Read the model definition and answer for the solid it produces. Units are mm, in the model's axes. A direction names the side the tool comes from. Round coordinates to 2 decimals unless told otherwise and drop trailing zeros. Write each loop counter-clockwise with the first axis right and the second up, starting at its lowest first coordinate (ties: lowest second). Pieces come first, ordered by that corner, then holes. Notation, with made-up numbers: (28, 56.25) - (39, 56.25) arc R29 cw to (39, 81.25) - close; hole circle Ø7 at (-14, 82). An arc over 180 degrees is marked (long way). Answer as CSV lines item,"result". Start each with the question number.
1) Find section C-C on y = -10. Determine the outline of the cut face in (x, z).
2) Find section B-B on z = 14.75. Determine the outline of the cut face in (x, y), then the cut area to 3 significant figures.
3) Find section D-D on x = -8.5. Determine the outline of the cut face in (y, z), then the cut area to 3 significant figures.
4) Find section A-A on z = 8.5. Determine the outline of the cut face in (x, y), then the cut area to 3 significant figures.
5) For a pull along Y with two mould halves and no side action, classify faces 3 (the flat face through (-26, -12.186, 8)), 4 (the cylindrical face through (-26.3, -3.58, 10.36)), 5 (the flat face through (-26, 10, 0)) as +Y half, -Y half, draft (parallel to the pull), parting line (faces both ways), or undercut.
6) Consider line 1 along X through (y, z) = (17, 8); line 2 along X through (y, z) = (-2, 9.5); line 3 along Y through (x, z) = (-0.5, 9.5). Determine where each line is inside the solid, lowest interval first.
7) Each of these flat-tipped pins is pushed along its axis until it touches: pin 1 (1 mm diameter, centred on y = 3.5, z = 4.5, fed in from +X); pin 2 (4.5 mm diameter, centred on x = -5.28, z = 8, fed in from -Y); pin 3 (12 mm diameter, centred on x = -7, y = 5, fed in from +Z) (1 decimal); pin 4 (6.5 mm diameter, centred on y = -4.18, z = 8.45, fed in from -X). Where does it stop, or does it pass through?
8) Which of the six approach directions +Z, -Z, +X, -X, +Y, -Y give full straight-line access (tool end or side, diameter ignored) to faces 1 (the flat face through (-12, 17.814, 8)), 2 (the flat face through (-11, 15.814, 8))?
from build123d import *

# Parameters (mm, degrees)
EXTRUDE_1_DEPTH     = 16
SKETCH_2_R          = 2
CUT_EXTRUDE_1_DEPTH = 16
SKETCH_3_R          = 2
CUT_EXTRUDE_2_DEPTH = 16


with BuildPart() as part:
    # 草图1 → 凸台-拉伸1 (new body)
    with BuildSketch(Plane.XY):
        Polygon((-27.281673393, 17.814060708), (-27.281673393, -12.185939292), (-25.281673393, -12.185939292), (-25.281673393, 15.814060708), (2.718326607, 15.814060708), (2.718326607, 17.814060708), align=None)
    extrude(amount=EXTRUDE_1_DEPTH)

    # 草图2 → 切除-拉伸1 (cut)
    with BuildSketch(Plane(origin=(0, 17.814060708, 0), x_dir=(1, 0, 0), z_dir=(0, 1, 0))):
        with Locations((-5.281673393, -8)):
            Circle(SKETCH_2_R)
    extrude(amount=-CUT_EXTRUDE_1_DEPTH, mode=Mode.SUBTRACT)

    # 草图3 → 切除-拉伸2 (cut)
    with BuildSketch(Plane.ZY.offset(27.281673393)):
        with Locations((8.454389853, -4.181246288)):
            Circle(SKETCH_3_R)
    extrude(amount=-CUT_EXTRUDE_2_DEPTH, mode=Mode.SUBTRACT)


solid = part.part
Check values:
1,outline,"(-27.28, 0) - (-25.28, 0) - (-25.28, 16) - (-27.28, 16) - close"
2,outline,"(-27.28, -12.19) - (-25.28, -12.19) - (-25.28, 15.81) - (2.72, 15.81) - (2.72, 17.81) - (-27.28, 17.81) - close"
2,area,"116 mm^2"
3,outline,"(15.81, 0) - (17.81, 0) - (17.81, 16) - (15.81, 16) - close"
3,area,"32.0 mm^2"
4,outline,"(-27.28, -12.19) - (-25.28, -12.19) - (-25.28, -6.18) - (-27.28, -6.18) - close; (-27.28, -2.18) - (-25.28, -2.18) - (-25.28, 15.81) - (-7.22, 15.81) - (-7.22, 17.81) - (-27.28, 17.81) - close; (-3.35, 15.81) - (2.72, 15.81) - (2.72, 17.81) - (-3.35, 17.81) - close"
4,area,"100 mm^2"
5,face 3,"-Y half"
5,face 4,"undercut"
5,face 5,"draft"
6,line 1,"x = -27.28 to -7.28, -3.28 to 2.72"
6,line 2,"x = -27.28 to -25.28"
6,line 3,"y = 15.81 to 17.81"
7,pin 1,"stops at x = -25.28"
7,pin 2,"stops at y = 15.81"
7,pin 3,"passes through"
7,pin 4,"stops at x = -27.28"
8,face 1,"+Z, -Z, +X, -X, +Y"
8,face 2,"+Z, -Z, +X, -Y"
